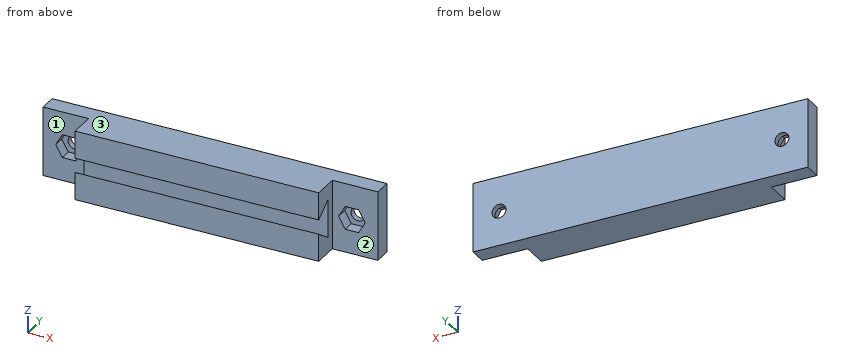
from build123d import *

# Parameters (mm, degrees)
SKETCH_1_W          = 42.2
SKETCH_1_H          = 12
EXTRUDE_1_DEPTH     = 6
CUT_EXTRUDE_1_DEPTH = 44.044628004
SKETCH_3_W          = 58
SKETCH_3_H          = 12
EXTRUDE_2_DEPTH     = 1.5
CUT_EXTRUDE_2_DEPTH = 2
CUT_EXTRUDE_3_REACH = 32.319
SKETCH_5_R          = 1.2


with BuildPart() as part:
    # 草图1 → 凸台-拉伸1 (new body)
    with BuildSketch(Plane(origin=(0, 0, 0), x_dir=(1, 0, 0), z_dir=(0, 1, 0))):
        Rectangle(SKETCH_1_W, SKETCH_1_H)
    extrude(amount=EXTRUDE_1_DEPTH)

    # 草图2 → 切除-拉伸1 (cut, through all)
    with BuildSketch(Plane(origin=(21.1, 0, 0), x_dir=(0, 0, -1), z_dir=(1, 0, 0))):
        Polygon((3.25, 3), (1.25, 0), (-1.25, 0), (-3.25, 3), align=None)
    extrude(amount=-CUT_EXTRUDE_1_DEPTH, mode=Mode.SUBTRACT)

    # 草图3 → 凸台-拉伸2 (add, symmetric)
    with BuildSketch(Plane(origin=(0, 6, 0), x_dir=(1, 0, 0), z_dir=(0, 1, 0))):
        Rectangle(SKETCH_3_W, SKETCH_3_H)
    extrude(amount=EXTRUDE_2_DEPTH, both=True)

    # 草图4 → 切除-拉伸2 (cut)
    with BuildSketch(Plane.XZ.offset(-4.5)):
        Polygon((-22.190598923, 0), (-23.345299462, 2), (-25.654700538, 2), (-26.809401077, 0), (-25.654700538, -2), (-23.345299462, -2), align=None)
        Polygon((22.190598923, 0), (23.345299462, 2), (25.654700538, 2), (26.809401077, 0), (25.654700538, -2), (23.345299462, -2), align=None)
    extrude(amount=-CUT_EXTRUDE_2_DEPTH, mode=Mode.SUBTRACT)

    # 草图5 → 切除-拉伸3 (cut, up to next)
    with BuildSketch(Plane.XZ.offset(-6.5), mode=Mode.PRIVATE) as cut_extrude_3_sk1:
        with Locations(Location((-24.5, 0, 0), (0, 0, 270))):
            Circle(SKETCH_5_R)
    cut_extrude_3_tool1 = extrude(cut_extrude_3_sk1.sketch, amount=-CUT_EXTRUDE_3_REACH, mode=Mode.PRIVATE) & part.part
    # 草图5 → 切除-拉伸3 (cut, up to next)
    with BuildSketch(Plane.XZ.offset(-6.5), mode=Mode.PRIVATE) as cut_extrude_3_sk2:
        with Locations(Location((24.5, 0, 0), (0, 0, 270))):
            Circle(SKETCH_5_R)
    cut_extrude_3_tool2 = extrude(cut_extrude_3_sk2.sketch, amount=-CUT_EXTRUDE_3_REACH, mode=Mode.PRIVATE) & part.part
    add(cut_extrude_3_tool1.solids().sort_by_distance((-24.5, 6.5, 0))[0], mode=Mode.SUBTRACT)
    add(cut_extrude_3_tool2.solids().sort_by_distance((24.5, 6.5, 0))[0], mode=Mode.SUBTRACT)


solid = part.part
Check sheet for the modelled part. Datum: model origin and axes. Units: mm. Face numbers are marked on the shaded views. A direction names the side the tool comes from. Give positions to 0.01 mm unless a question says otherwise; leave off trailing zeros. Loops run counter-clockwise (first coordinate to the right, second up) from the corner with the lowest first, then second, coordinate; pieces in that order, holes last. Notation, with made-up numbers: M -37.5,9 L 8.5,9 A14 ccw 8.5,13 Z; hole C 26.25,74 d8. An arc over 180 degrees is marked long. Answer as a JSON object with one key per item and string values. Group by question number.
Q1. Cross-section at C-C on x = -17.5. Record the cut outline in (y, z).
Q2. Cross-section at B-B on y = 2.25. Record the cut outline in (x, z).
Q3. Cross-section at A-A on x = -24.5. Record the cut outline in (y, z).
Q4. Go/stop test with flat-tipped pins: P1, Ø4.5, axis at x = -25, z = 0, coming from the -Y side; P2, Ø3.5, axis at y = 2.5, z = -1.5, coming from the -X side; P3, Ø3, axis at y = 1, z = 2.5, coming from the +X side. Record where each tip stops, or that it passes through.
Q5. Material ranges on line 1 along X through (y, z) = (7.3, 0); line 2 along Y through (x, z) = (-25, -4.75); line 3 along X through (y, z) = (2.25, -4.5), recorded low to high. Write a range as [from, to].
Q6. Access from +Z, -Z, +X, -X, +Y, -Y to the whole of each face (thin tool, end or side, straight path). Record for the marked faces 1, 2 and 3.
Evaluation:
{
 "1": {"outline": "M 0,-6 L 7.5,-6 L 7.5,6 L 0,6 L 0,1.25 L 3,3.25 L 3,-3.25 L 0,-1.25 Z"},
 "2": {"outline": "M -21.1,-6 L 21.1,-6 L 21.1,-2.75 L -21.1,-2.75 Z; M -21.1,2.75 L 21.1,2.75 L 21.1,6 L -21.1,6 Z"},
 "3": {"outline": "M 4.5,-6 L 7.5,-6 L 7.5,-1.2 L 6.5,-1.2 L 6.5,-2 L 4.5,-2 Z; M 4.5,2 L 6.5,2 L 6.5,1.2 L 7.5,1.2 L 7.5,6 L 4.5,6 Z"},
 "4": {"P1": "stops at y = 4.5", "P2": "stops at x = -21.1", "P3": "stops at x = 21.1"},
 "5": {"line 1": "x = [-29, -25.7], [-23.3, 23.3], [25.7, 29]", "line 2": "y = [4.5, 7.5]", "line 3": "x = [-21.1, 21.1]"},
 "6": {"face 1": "+Z, -Z, -X, -Y", "face 2": "+Z, -Z, +X, -Y", "face 3": "+Z, +X, -X, +Y, -Y"}
}
